Verification items for the finished model (mm, model axes). A direction names the side the tool comes from. Coordinates: 2 decimals unless noted, no trailing zeros. Order: outer loops, then holes, each group sorted by start corner. A loop starts at its lowest first (then second) coordinate and runs counter-clockwise, first axis right, second up.
Q1. Set-up check for faces 1 (the flat face through (-291, 1, 65)), 2 (the cylindrical face through (299.54, 3, 31.34)): record each of +Z, -Z, +X, -X, +Y, -Y from which the full face is reachable in a straight line by a thin tool's end or side.
Q2. Draft check along X on faces 3 (the cylindrical face through (-280.46, 3, 31.34)), 4 (the cylindrical face through (359.28, -28.73, 52.32)), 5 (the cylindrical face through (4.614, -298.872, 31.336)), 6 (the flat face through (16, -289, 40)). Enter one of: pulls with the +X half, pulls with the -X half, needs draft (parallel to the pull), parting line crosses it, or undercut.
Q3. Depth check by flat-ended pin: P1, Ø5, axis at x = 17, y = 45, coming from the -Z side; P2, Ø12, axis at x = 16.5, y = -36, coming from the +Z side; P3, Ø1.5, axis at x = -170.5, z = -6, coming from the +Y side. Enter the tip coordinate at first touch or a pass-through.
Q4. Cross-section at B-B, the plane z = -9. Record the boundary of the cut face in (x, y), and give its area (3 significant figures).
Q5. Cross-section at A-A, the plane x = -51.5. Record the boundary of the cut face in (y, z), and give its area (3 significant figures).
Q6. Thickness scan on line 1 (Z direction, x = 36, y = -317.5); line 2 (Z direction, x = 21.5, y = 255); line 3 (Y direction, x = 48.5, z = -14). Record the ranges inside material, lowest first.
Q7. Cross-section at C-C, the plane y = 135.5. Record the boundary of the cut face in (x, z), and give its area (3 significant figures).
from build123d import *

# Parameters (mm, degrees)
F0_R     = 25
F1_DEPTH = 320
F2_COUNT = 2
F2_ANGLE = 90
F3_R     = 25
F4_R     = 10
F5_DEPTH = 40
F7_R     = 75
F8_DEPTH = 25


with BuildPart() as f1:
    # F0 (on Front) → F1 (new body, symmetric)
    with BuildSketch(Plane.XZ):
        Circle(F0_R)
    extrude(amount=F1_DEPTH, both=True)

    # F2: F1 ×2 about axis
    f2_axis = Axis((0, 0, 1.4691501971), (0, 0, -1))


with BuildPart() as f1_1:
    add(f1.part)
    for i in range(1, F2_COUNT):
        add(f1.part.rotate(f2_axis, i * F2_ANGLE / (F2_COUNT - 1)))

    # F3
    f3_edges = [f1_1.edges().sort_by_distance(p)[0] for p in [
        (-25, -320, 0),
        (320, 25, 0),
        (-25, 320, 0),
        (-320, 25, 0),
    ]]
    fillet(f3_edges, radius=F3_R)

    # F4 (on Top) → F5 (join)
    with BuildSketch(Plane.XY):
        with Locations((-290, 0)):
            Circle(F4_R)
        with Locations((0, -290)):
            Circle(F4_R)
        with Locations((290, 0)):
            Circle(F4_R)
        with Locations((0, 290)):
            Circle(F4_R)
    extrude(amount=F5_DEPTH)

    # F7 (on offset) → F8 (join)
    with BuildSketch(Plane.XY.offset(40)):
        with Locations((-290, 0)):
            Circle(F7_R)
        with Locations((-3.72e-08, 290)):
            Circle(F7_R)
        with Locations((290, 7.44e-08)):
            Circle(F7_R)
        with Locations((1.116e-07, -290)):
            Circle(F7_R)
    extrude(amount=F8_DEPTH)


solid = f1_1.part
Check values:
1. face 1: +Z, +X, -X, +Y, -Y
1. face 2: none
2. face 3: undercut
2. face 4: undercut
2. face 5: parting line crosses it
2. face 6: needs draft
3. P1: stops at z = -20.37
3. P2: stops at z = 22.69
3. P3: stops at y = 24.44
4. outline: (-295, -23.32) - (-23.32, -23.32) - (-23.32, -295) arc R23.32 ccw to (23.32, -295) - (23.32, -23.32) - (295, -23.32) arc R23.32 ccw to (295, 23.32) - (23.32, 23.32) - (23.32, 295) arc R23.32 ccw to (-23.32, 295) - (-23.32, 23.32) - (-295, 23.32) arc R23.32 ccw to start
4. area: 56,300 mm2
5. outline: (-344.52, 40) - (-235.48, 40) - (-235.48, 65) - (-344.52, 65) - close; circle Ø50 at (0, 0); (235.48, 40) - (344.52, 40) - (344.52, 65) - (235.48, 65) - close
5. area: 7,420 mm2
6. line 1: z = 40 to 65
6. line 2: z = -12.76 to 12.76, 40 to 65
6. line 3: y = -20.71 to 20.71
7. outline: circle Ø50 at (0, 0)
7. area: 1,960 mm2
